from build123d import *

# Parameters (mm, degrees)
SKETCH1_R               = 22.5
BOSS_EXTRUDE1_DEPTH     = 3
SKETCH2_R               = 5
BOSS_EXTRUDE2_DEPTH     = 70
SKETCH3_R               = 12
BOSS_EXTRUDE3_DEPTH     = 28
FILLET1_R               = 6
CUT_EXTRUDE1_DEPTH      = 80.633535649
CUT_EXTRUDE1_DEPTH_BACK = 80.633535649
SKETCH4_W               = 15.997747603
SKETCH4_H               = 20
SKETCH5_R               = 4
CUT_EXTRUDE2_DEPTH      = 83.068568892
SKETCH6_R               = 9
SKETCH6_R_2             = 4
BOSS_EXTRUDE15_DEPTH    = 3.5
SKETCH10_R              = 9
SKETCH10_R_2            = 4
BOSS_EXTRUDE19_DEPTH    = 3


with BuildPart() as part:
    # Sketch1 → Boss-Extrude1 (new body)
    with BuildSketch(Plane(origin=(0, 0, 0), x_dir=(1, 0, 0), z_dir=(0, 1, 0))):
        with Locations(Location((0, 0, 0), (0, 0, 270))):
            Circle(SKETCH1_R)
    extrude(amount=BOSS_EXTRUDE1_DEPTH)

    # Sketch2 → Boss-Extrude2 (add)
    with BuildSketch(Plane(origin=(0, 3, 0), x_dir=(1, 0, 0), z_dir=(0, 1, 0))):
        with Locations(Location((0, 0, 0), (0, 0, 270))):
            Circle(SKETCH2_R)
    extrude(amount=BOSS_EXTRUDE2_DEPTH)

    # Sketch3 → Boss-Extrude3 (add)
    with BuildSketch(Plane.XZ):
        with Locations(Location((0, 0, 0), (0, 0, 270))):
            Circle(SKETCH3_R)
    extrude(amount=BOSS_EXTRUDE3_DEPTH)

    # Fillet1
    fillet1_edges = [part.edges().sort_by_distance(p)[0] for p in [
        (0, -28, 12),
    ]]
    fillet(fillet1_edges, radius=FILLET1_R)

    # Sketch4 → Cut-Extrude1 (cut, two sides: drawn at the far end of the back side and taken through both)
    with BuildSketch(Plane.XY.offset(-CUT_EXTRUDE1_DEPTH_BACK)):
        with Locations((-15.498873802, -17.840930737)):
            Rectangle(SKETCH4_W, SKETCH4_H)
        with Locations((15.498873802, -17.840930737)):
            Rectangle(SKETCH4_W, SKETCH4_H)
    extrude(amount=CUT_EXTRUDE1_DEPTH + CUT_EXTRUDE1_DEPTH_BACK, mode=Mode.SUBTRACT)

    # Sketch5 → Cut-Extrude2 (cut, through all)
    with BuildSketch(Plane(origin=(7.5, 0, 0), x_dir=(0, 0, -1), z_dir=(1, 0, 0))):
        with Locations(Location((0, -18, 0), (0, 0, 90))):
            Circle(SKETCH5_R)
    extrude(amount=-CUT_EXTRUDE2_DEPTH, mode=Mode.SUBTRACT)

    # Sketch6 → Boss-Extrude15 (add, symmetric)
    with BuildSketch(Plane(origin=(7.5, 0, 0), x_dir=(0, 0, -1), z_dir=(1, 0, 0))):
        with Locations(Location((0, -18, 0), (0, 0, 270))):
            Circle(SKETCH6_R)
        with Locations(Location((0, -18, 0), (0, 0, 90))):
            Circle(SKETCH6_R_2, mode=Mode.SUBTRACT)
    extrude(amount=BOSS_EXTRUDE15_DEPTH, both=True)

    # Sketch10 → Boss-Extrude19 (add)
    with BuildSketch(Plane.ZY.offset(7.5)):
        with Locations(Location((0, -18, 0), (0, 0, 270))):
            Circle(SKETCH10_R)
        with Locations(Location((0, -18, 0), (0, 0, 90))):
            Circle(SKETCH10_R_2, mode=Mode.SUBTRACT)
    extrude(amount=BOSS_EXTRUDE19_DEPTH)


solid = part.part
Geometry check sheet. Reference: the model listing, model coordinates, mm. A direction names the side the tool comes from. Give positions to 0.01 mm unless a question says otherwise; leave off trailing zeros. Write each loop counter-clockwise with the first axis right and the second up, starting at its lowest first coordinate (ties: lowest second). Pieces come first, ordered by that corner, then holes.
1) Go/stop test with flat-tipped pins: pin 1 Ø3 at (y, z) = (60.5, -2.5) entering from -X; pin 2 Ø20 at (y, z) = (-20.5, -2) entering from -X; pin 3 Ø10 at (x, y) = (8.5, 35.5) entering from -Z. Record where each tip stops, or that it passes through.
Values follow:
pin 1: stops at x = -4.9
pin 2: stops at x = -10.5
pin 3: stops at z = -3.57
2) Set-up check for faces 1 (the face through (9.275, -26.584, -2.703)), 2 (the face through (-7.5, -9, 2)), 3 (the face through (11, -22, 2)): record each of +Z, -Z, +X, -X, +Y, -Y from which the full face is reachable in a straight line by a thin tool's end or side.
Values follow:
face 1: +X
face 2: -X
face 3: +Z, -Z, +X, -Y
3) Release check for a two-part mould opening along Z. For faces 4 (the face through (0.4, -21.2, 2.4)), 5 (the face through (5.3, 3, -0.3)), 6 (the face through (-11.715, -5.957, 2.601)) record: released by +Z, released by -Z, zero draft, split by the parting line, or undercut.
Values follow:
face 4: undercut
face 5: zero draft
face 6: split by the parting line
4) Thickness scan on line 1 (Y direction, x = -3, z = 0); line 2 (Y direction, x = 6, z = 0); line 3 (Y direction, x = -7.5, z = -11). Record the ranges inside material, lowest first.
Values follow:
line 1: y = -28 to -22, -14 to 73
line 2: y = -28 to -22, -14 to 3
line 3: y = 0 to 3
5) Cross-section at A-A (y = -18). Record the boundary of the cut face in (x, z), plus the area to 3 significant figures.
Values follow:
outline: (-10.5, -9) - (-7.5, -9) - (-7.5, -9.37) arc R12 ccw to (7.5, -9.37) - (7.5, -9) - (11, -9) - (11, -4) - (-10.5, -4) - close; (-10.5, 4) - (11, 4) - (11, 9) - (7.5, 9) - (7.5, 9.37) arc R12 ccw to (-7.5, 9.37) - (-7.5, 9) - (-10.5, 9) - close
area: 280 mm2
6) Cross-section at D-D (z = 19). Record the boundary of the cut face in (x, y), plus the area to 3 significant figures.
Values follow:
outline: (-12.05, 0) - (12.05, 0) - (12.05, 3) - (-12.05, 3) - close
area: 72.3 mm2
7) Cross-section at C-C (x = -14.5). Record the boundary of the cut face in (y, z), plus the area to 3 significant figures.
Values follow:
outline: (0, -17.2) - (3, -17.2) - (3, 17.2) - (0, 17.2) - close
area: 103 mm2
8) Cross-section at B-B (y = -1.5). Record the boundary of the cut face in (x, z), plus the area to 3 significant figures.
Values follow:
outline: circle Ø24 at (0, 0)
area: 452 mm2
